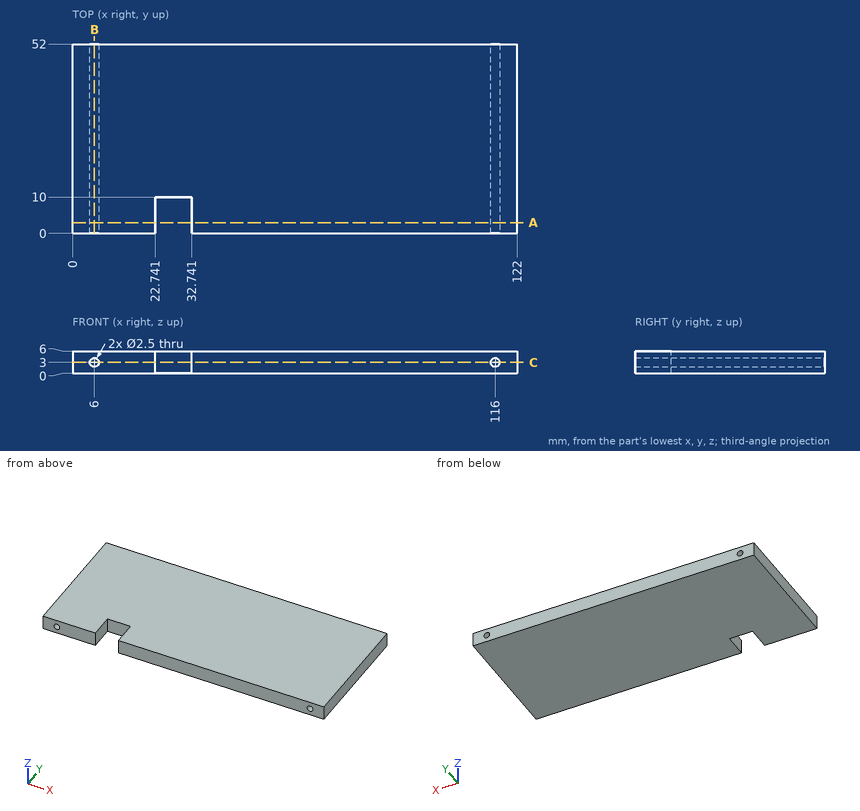
Here's the drawing with two shaded views (mm, measured from the low corner). I have some questions. Coordinates: 2 decimals unless noted, no trailing zeros. Loops run counter-clockwise (first coordinate to the right, second up) from the corner with the lowest first, then second, coordinate; pieces in that order, holes last. Notation, with made-up numbers: (76, -28) -> (84, -28) arc R22 cw to (84, 1) -> close; hole circle Ø4 at (34.25, -39). An arc over 180 degrees is marked (long way). Answer in a Markdown table with one row per item.
(1) Imagine slicing it at C-C (z = 3). List the corners of the cut face in (x, y) for me, plus the area to 3 significant figures.
Results found:
| item | result |
|---|---|
| outline | (0, 0) -> (4.75, 0) -> (4.75, 52) -> (0, 52) -> close; (7.25, 0) -> (22.74, 0) -> (22.74, 10) -> (32.74, 10) -> (32.74, 0) -> (114.75, 0) -> (114.75, 52) -> (7.25, 52) -> close; (117.25, 0) -> (122, 0) -> (122, 52) -> (117.25, 52) -> close |
| area | 5,980 mm^2 |
(2) Imagine slicing it at A-A (y = 3). List the corners of the cut face in (x, z) for me, plus the area to 3 significant figures.
Results found:
| item | result |
|---|---|
| outline | (0, 0) -> (22.74, 0) -> (22.74, 6) -> (0, 6) -> close; (32.74, 0) -> (122, 0) -> (122, 6) -> (32.74, 6) -> close; hole circle Ø2.5 at (6, 3); hole circle Ø2.5 at (116, 3) |
| area | 662 mm^2 |
(3) If I drill on probe 1 along X at (y, z) = (29.5, 3); probe 2 along Z at (x, y) = (116, 37.5); probe 3 along X at (y, z) = (19, 2), over which ranges is the centre line in solid material (lowest first)?
Results found:
| item | result |
|---|---|
| probe 1 | x = 0 to 4.75, 7.25 to 114.75, 117.25 to 122 |
| probe 2 | z = 0 to 1.75, 4.25 to 6 |
| probe 3 | x = 0 to 5.25, 6.75 to 115.25, 116.75 to 122 |
(4) Will these pins go through, and if not, where does the flat tip stop? pin 1 Ø3 at (x, z) = (116, 3) entering from -Y; pin 2 Ø3 at (x, z) = (26, 3) entering from -Y.
Results found:
| item | result |
|---|---|
| pin 1 | stops at y = 0 |
| pin 2 | stops at y = 10 |
(5) Imagine slicing it at B-B (x = 6). List the corners of the cut face in (y, z) for me.
Results found:
| item | result |
|---|---|
| outline | (0, 0) -> (52, 0) -> (52, 1.75) -> (0, 1.75) -> close; (0, 4.25) -> (52, 4.25) -> (52, 6) -> (0, 6) -> close |
